Input: part model. Units: mm. Frame: model coordinates. A direction names the side the tool comes from. Coordinates: 2 decimals unless noted, no trailing zeros. Write each loop counter-clockwise with the first axis right and the second up, starting at its lowest first coordinate (ties: lowest second). Pieces come first, ordered by that corner, then holes. Notation, with made-up numbers: M 9,67 L 29,67 A21 cw 29,82 Z; hole C -37.75,42 d8. An arc over 180 degrees is marked long. Write each question's results on one line, items separated by ' | '. Start each with the question number.
1. Section query D-D, the plane z = 5.25. Output: boundary loops of the cut face in (x, y).
2. First-contact query: pin 1 (3 mm diameter, centred on y = 7, z = 2.5, fed in from +X); pin 2 (2.5 mm diameter, centred on x = 15, z = 5, fed in from -Y); pin 3 (3 mm diameter, centred on x = 6.5, y = 6.5, fed in from +Z); pin 4 (2 mm diameter, centred on x = 17, z = 6.5, fed in from +Y). Flat tips, straight axial feed; report the tip coordinate or a pass-through.
3. Section query B-B, the plane y = 4. Output: boundary loops of the cut face in (x, z).
4. Ray query, probe 1 along Z at (x, y) = (15, 1.85); probe 2 along Y at (x, z) = (5, 1.45); probe 3 along Z at (x, y) = (6.5, 8). Return the intervals inside material, ascending.
5. Set-up query: faces 4 (the flat face through (7, 5, 2)), 5 (the flat face through (0, 5, 1)), 6 (the flat face through (10, 7, 1)). Return all of +Z, -Z, +X, -X, +Y, -Y with unobstructed straight access to the full face (end or side cutting, diameter ignored); none if empty.
6. Pull-direction query (X, two-part tool) for faces 1 (the flat face through (11.5, 0, 3.6)), 2 (the cylindrical face through (13.5, 2.46, 5.07)), 3 (the flat face through (19, 2, 3)); classes: +X half, -X half, draft (parallel to the pull), parting line (faces both ways), or undercut.
7. Section query C-C, the plane y = 1.75. Output: boundary loops of the cut face in (x, z), and give its area (3 significant figures).
8. Section query A-A, the plane x = 5. Output: boundary loops of the cut face in (y, z).
```python
from build123d import *

# Parameters (mm, degrees)
ESQUISSE1_R        = 1.5
BOSS_EXTRU_2_DEPTH = 2
ESQUISSE4_R        = 1.5
BOSS_EXTRU_3_DEPTH = 5


with BuildPart() as part:
    # Esquisse1 → Boss.-Extru.2 (new body)
    with BuildSketch(Plane.XY):
        Polygon((0, 0), (15, 0), (15, 5), (10, 5), (10, 10), (0, 10), align=None)
        with Locations((5, 5)):
            Circle(ESQUISSE1_R, mode=Mode.SUBTRACT)
    extrude(amount=BOSS_EXTRU_2_DEPTH)

    # Esquisse4 → Boss.-Extru.3 (add)
    with BuildSketch(Plane.XZ):
        with BuildLine():
            Line((11, 5), (11, 0))
            Line((11, 0), (15.535898385, 0))
            ThreePointArc((15.535898385, 0), (17.535898385, 0.535898385), (19, 2))
            Line((19, 2), (19, 5))
            ThreePointArc((19, 5), (15, 9), (11, 5))
        make_face()
        with Locations((15, 5)):
            Circle(ESQUISSE4_R, mode=Mode.SUBTRACT)
    extrude(amount=-BOSS_EXTRU_3_DEPTH)


solid = part.part
```
Answer:
1) outline: M 11.01,0 L 13.52,0 L 13.52,5 L 11.01,5 Z; M 16.48,0 L 18.99,0 L 18.99,5 L 16.48,5 Z
2) pin 1: x = 10 | pin 2: through | pin 3: z = 2 | pin 4: y = 5
3) outline: M 0,0 L 3.88,0 L 3.88,2 L 0,2 Z; M 6.12,0 L 15.54,0 A4 ccw 19,2 L 19,5 A4 ccw 11,5 L 11,2 L 6.12,2 Z; hole C 15,5 d3
4) probe 1: 0 to 3.5, 6.5 to 9 | probe 2: 0 to 3.5, 6.5 to 10 | probe 3: 0 to 2
5) face 4: +Z, -X, +Y, -Y | face 5: +Z, -Z, -X, +Y, -Y | face 6: +Z, -Z, +X, +Y
6) face 1: draft | face 2: undercut | face 3: +X half
7) outline: M 0,0 L 15.54,0 A4 ccw 19,2 L 19,5 A4 ccw 11,5 L 11,2 L 0,2 Z; hole C 15,5 d3 | area: 78.0 mm^2
8) outline: M 0,0 L 3.5,0 L 3.5,2 L 0,2 Z; M 6.5,0 L 10,0 L 10,2 L 6.5,2 Z
